Part model, mm, in its own coordinate system. A direction names the side the tool comes from. Round coordinates to 2 decimals unless told otherwise and drop trailing zeros. One line per question, with ' | ' between items. Start each with the question number.
1) Tool access for faces 4 (the face through (7, -7, 55)), 5 (the face through (12, -11, 30)), 6 (the face through (4.2, -7, 23)): list every direction of +Z, -Z, +X, -X, +Y, -Y with a clear straight run to the whole face (end or side of a thin tool).
2) Wall check: probe 1 along X at (y, z) = (-10.5, 38.5); probe 2 along X at (y, z) = (-3, 33); probe 3 along Y at (x, z) = (11.25, 35.5). Give the ranges that are in metal, low to high. Write a range as [from, to].
3) Drop a flat-ended pin along its axis: pin 1 Ø3 at (y, z) = (-6, 53) entering from -X. Give the stop position or say it passes through.
4) Mould opens along Y. For faces 1 (the face through (9, -14.8, 30)), 2 (the face through (6, -6, 49)), 3 (the face through (11, 0, 30)) say: pulls with the +Y half, pulls with the -Y half, needs draft (parallel to the pull), parting line crosses it, or undercut.
Autodesk Inventor part; units mm, degrees
ref_plane "YZ Plane" through (0, 0, 0) normal (1, 0, 0) x (0, 1, 0)
ref_plane "XZ Plane" through (0, 0, 0) normal (0, 1, 0) x (-1, 0, 0)
ref_plane "XY Plane" through (0, 0, 0) normal (0, 0, 1) x (1, 0, 0)
sketch "Sketch1" plane through (0, 0, 0) normal (0, 0, 1) x (1, 0, 0)
  arc A0 (16, 5) -> (14, 7) centre (14, 5) ccw
  line L0 (14, 7) -> (8, 7)
  arc A1 (6, 9) -> (8, 7) centre (8, 9) ccw
  line L1 (6, 9) -> (6, 25.5)
  arc A2 (6, 25.5) -> (4, 27.5) centre (4, 25.5) ccw
  line L2 (4, 27.5) -> (-14, 27.5)
  arc A3 (-14, 27.5) -> (-16, 25.5) centre (-14, 25.5) ccw
  line L3 (-16, 25.5) -> (-16, 20.5)
  line L4 (-16, 20.5) -> (4, 20.5)
  line L5 (4, 20.5) -> (4, 5)
  line L6 (4, 5) -> (14, 5)
  line L7 (14, 5) -> (14, -15)
  line L8 (14, -15) -> (4, -15)
  line L9 (4, -15) -> (4, -20.5)
  line L10 (4, -20.5) -> (-16, -20.5)
  line L11 (-16, -20.5) -> (-16, -25.5)
  arc A4 (-16, -25.5) -> (-14, -27.5) centre (-14, -25.5) ccw
  line L12 (-14, -27.5) -> (4, -27.5)
  arc A5 (4, -27.5) -> (6, -25.5) centre (4, -25.5) ccw
  line L13 (6, -25.5) -> (6, -19)
  arc A6 (8, -17) -> (6, -19) centre (8, -19) ccw
  line L14 (8, -17) -> (14, -17)
  arc A7 (14, -17) -> (16, -15) centre (14, -15) ccw
  line L15 (16, -15) -> (16, 5)
  circle A8 centre (-10.2273, -23.9687) radius 0.75
  circle A9 centre (-0.7, 24) radius 0.75
  circle A10 centre (-10.2, 24) radius 0.75
  circle A11 centre (-0.7, -24) radius 0.75
  line L16 (11.5, 0) -> (9.5, 0)
  line L17 (9.5, -13) -> (11.5, -13)
  line L18 (12.5, -11) -> (12.5, -7)
  line L19 (8.5, -7) -> (8.5, -11)
  line L20 (8.5, -11) -> (12.5, -7) construction
  line L21 (12.5, -11) -> (8.5, -7) construction
  line L22 (8.5, -11) -> (9.5, -11)
  line L23 (11.5, -11) -> (12.5, -11)
  line L24 (12.5, -7) -> (11.5, -7)
  line L25 (9.5, -7) -> (8.5, -7)
  line L26 (11.5, -13) -> (11.5, -11)
  line L27 (11.5, -7) -> (11.5, 0)
  line L28 (9.5, 0) -> (9.5, -7)
  line L29 (9.5, -11) -> (9.5, -13)
  line L30 (14, -15) -> (4, -15)
  line L31 (4, -15) -> (4, 2)
  line L32 (4, 2) -> (14, 2)
  line L33 (14, 2) -> (14, -15)
  point P0 (0, 0)
  point P1 (10.5, -9)
  dimension "d0" = 2
  dimension "d1" = 13
  dimension "d2" = 4
  dimension "d3" = 4
  dimension "d5" = 17
  dimension "d6" = 1.5
  dimension "d7" = 2
  dimension "d8" = 2
  dimension "d12" = 1
  dimension "d13" = 1
extrude "Extrusion1" add sketch "Sketch1" along normal blind 50 contours L31 L32 L7 L8
sketch "Sketch2" plane through (0, 0, 50) normal (0, 0, 1) x (1, 0, 0)
  line L0 (14, -15) -> (14, 2)
  line L1 (14, 2) -> (4, 2)
  line L2 (4, 2) -> (4, -15)
  line L3 (4, -15) -> (14, -15)
  line L4 (8.5, -7) -> (9.5, -7)
  line L5 (9.5, -7) -> (9.5, 0)
  line L6 (9.5, 0) -> (11.5, 0)
  line L7 (11.5, 0) -> (11.5, -7)
  line L8 (11.5, -7) -> (12.5, -7)
  line L9 (12.5, -7) -> (12.5, -11)
  line L10 (12.5, -11) -> (11.5, -11)
  line L11 (11.5, -11) -> (11.5, -13)
  line L12 (11.5, -13) -> (9.5, -13)
  line L13 (9.5, -13) -> (9.5, -11)
  line L14 (9.5, -11) -> (8.5, -11)
  line L15 (8.5, -11) -> (8.5, -7)
  line L16 (14, 2) -> (4, 2)
  line L17 (14, -15) -> (7, -15)
  line L18 (7, -15) -> (7, 2)
  line L19 (7, 2) -> (14, 2)
  line L20 (14, 2) -> (14, -15)
  point P0 (0, 0)
  point P1 (7, 2)
  dimension "d11" = 3
extrude "Extrusion2" add sketch "Sketch2" along normal blind 10 contours L3 L18 L1 L0
chamfer "Chamfer1" distance 3 angle 45 1 edges at (4, -6.5, 50)
thicken "Thicken1" operation add thickness 0.2 both sides no extend neighbours yes toward (1, 0, 0) faces at (4, -3.6667, 15.6667) (7.3333, -15, 15.6667) (7.3333, 2, 15.6667) (14, -9.3333, 20)
chamfer "Chamfer2" distance 1 angle 45 2 edges at (11.5, -7, 30) (9.5, -7, 30)
equation "\"d13\" = d12"
properties part number "funnel"
Answer key:
1) face 4: +Z, -X, +Y, -Y | face 5: +Z, -Z | face 6: +Z, -Z, -X, +Y, -Y
2) probe 1: x = [4.2, 8.5], [12.5, 13.8] | probe 2: x = [4.2, 9.5], [11.5, 13.8] | probe 3: y = [-14.8, -13], [0, 1.8]
3) pin 1: stops at x = 7
4) face 1: pulls with the -Y half | face 2: needs draft | face 3: undercut
